For this review, use the dimensioned drawing (mm, ordinates from the lowest corner) and the shaded views. Coordinates: 2 decimals unless noted, no trailing zeros. Write each loop counter-clockwise with the first axis right and the second up, starting at its lowest first coordinate (ties: lowest second). Pieces come first, ordered by that corner, then holes. Notation, with made-up numbers: M 38,25 L 88,25 A22 ccw 88,31 Z; hole C 64.5,-8.75 d6. An arc over 180 degrees is marked long. One line per question, with ' | ' between items.
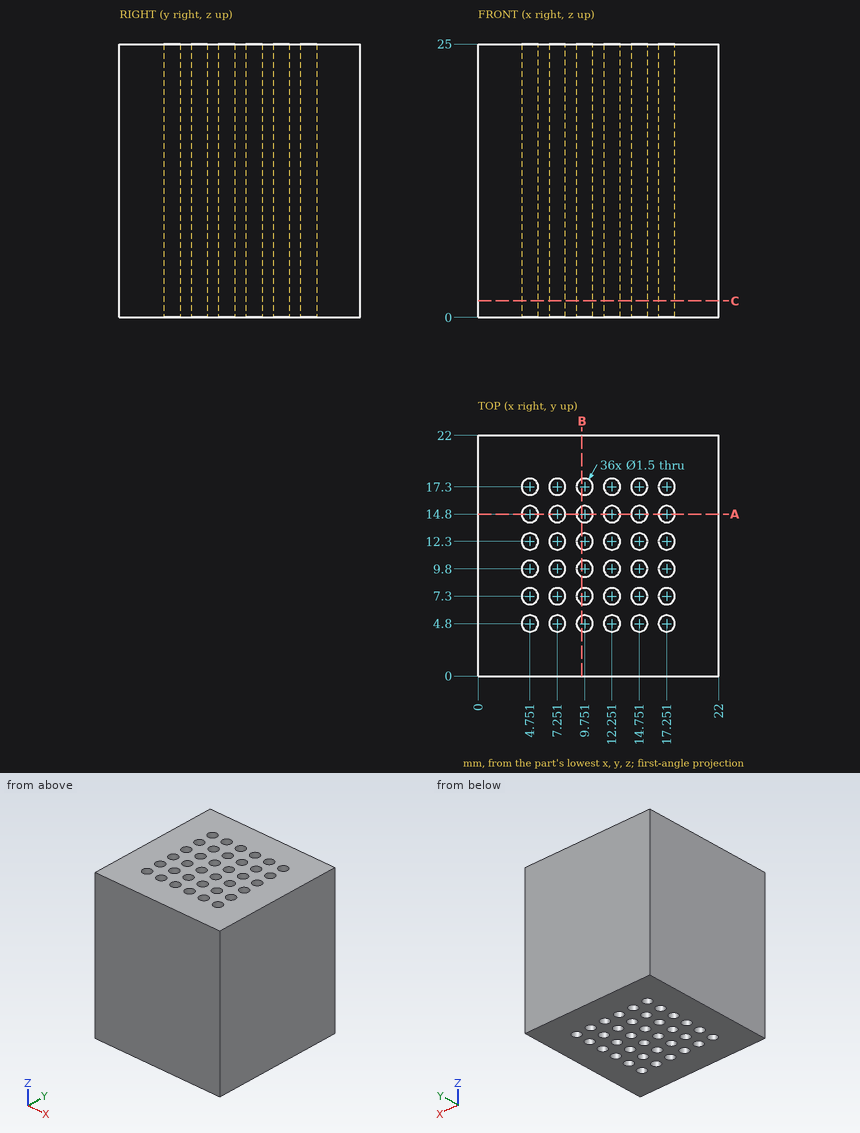
1) We need section A-A on y = 14.8. State the section outline as (x, z) points.
Responses:
outline: M 0,0 L 4,0 L 4,25 L 0,25 Z; M 5.5,0 L 6.5,0 L 6.5,25 L 5.5,25 Z; M 8,0 L 9,0 L 9,25 L 8,25 Z; M 10.5,0 L 11.5,0 L 11.5,25 L 10.5,25 Z; M 13,0 L 14,0 L 14,25 L 13,25 Z; M 15.5,0 L 16.5,0 L 16.5,25 L 15.5,25 Z; M 18,0 L 22,0 L 22,25 L 18,25 Z
2) We need section B-B on x = 9.5. State the section outline as (y, z) points.
Responses:
outline: M 0,0 L 4.09,0 L 4.09,25 L 0,25 Z; M 5.51,0 L 6.59,0 L 6.59,25 L 5.51,25 Z; M 8.01,0 L 9.09,0 L 9.09,25 L 8.01,25 Z; M 10.51,0 L 11.59,0 L 11.59,25 L 10.51,25 Z; M 13.01,0 L 14.09,0 L 14.09,25 L 13.01,25 Z; M 15.51,0 L 16.59,0 L 16.59,25 L 15.51,25 Z; M 18.01,0 L 22,0 L 22,25 L 18.01,25 Z
3) Insertion check: pin 1 Ø8 at (x, z) = (9, 17) entering from -Y; pin 2 Ø1.4 at (x, y) = (12.25, 7.3) entering from +Z. Each pin has a flat end and moves straight along its axis. Give the tip position at first contact, or say it passes through.
Responses:
pin 1: y = 0 | pin 2: through
4) We need section C-C on z = 1.5. State how many separate pieces and enclosed holes the cut face has.
Responses:
separate pieces: 1 | enclosed holes: 36
